Design review of the part built by this model. Coordinates are the model's own, in mm. A direction names the side the tool comes from. Round coordinates to 2 decimals unless told otherwise and drop trailing zeros. Order: outer loops, then holes, each group sorted by start corner. A loop starts at its lowest first (then second) coordinate and runs counter-clockwise, first axis right, second up. Notation, with made-up numbers: (8, 73.25) - (54, 73.25) arc R25 cw to (54, 103.25) - close; hole circle Ø8 at (-36, 74). An arc over 180 degrees is marked (long way). Use CSV: the item, a comma, the result in double quotes.
Autodesk Inventor part; units mm, degrees
ref_plane "XZ Plane" through (0, 0, 0) normal (0, 1, 0) x (-1, 0, 0)
ref_plane "XY Plane" through (0, 0, 0) normal (0, 0, 1) x (1, 0, 0)
sketch "Sketch1" plane through (0, 0, 0) normal (0, 1, 0) x (-1, 0, 0)
  circle A0 centre (0, 0) radius 17.5
  arc A1 (-20.1304, -3.875) -> (-20.1304, 3.875) centre (0, 0) ccw
  line L0 (-20.5, -3.875) -> (-20.5, -13.4374) construction
  line L1 (-20.5, -13.4374) -> (-20.5, 14.7091) construction
  line L2 (-47.5, 3.875) -> (-47.5, -3.875)
  line L3 (-47.5, -3.875) -> (-20.1304, -3.875)
  line L4 (0, 0) -> (-47.4736, 0) construction
  line L5 (-47.5, 3.875) -> (-20.1304, 3.875)
  dimension "d0" = 35
  dimension "d1" = 3
  dimension "d4" = 27
extrude "Extrusion1" add sketch "Sketch1" along normal blind 40
sketch "Sketch2" plane through (20.1304, 0, 3.875) normal (0, 0, 1) x (1, 0, 0)
  line L0 (27.3696, 0) -> (27.3696, 40)
  line L1 (2, 40) -> (27.3696, 40)
  line L2 (17.5718, 20.8426) -> (6, 0)
  line L3 (27.3696, 0) -> (0, 0)
  line L4 (27.3696, 0) -> (27.3696, 40)
  line L5 (6, 0) -> (27.3696, 0)
  line L6 (27.3696, 0) -> (27.3696, 28)
  line L7 (0, 0) -> (0, 40)
  arc A0 (17.5718, 20.8426) -> (12.9208, 36.4588) centre (17, 29.173) ccw
  line L8 (12.9208, 36.4588) -> (0, 40)
  circle A1 centre (17, 29.173) radius 3.825
  line L9 (0, 40) -> (27.3696, 40)
  line L10 (27.3696, 0) -> (6, 0)
  point P0 (-20.1304, 0)
  dimension "d10" = 6
  dimension "d14" = 16.7
  dimension "d15" = 17
  dimension "d16" = 7.65
extrude "Extrusion2" cut sketch "Sketch2" against normal blind 40 contours L3 L2 A0 L8 L9 L1 L0 | A1
ref_plane "Work Plane1" through (-12, 0, 0) normal (1, 0, 0) x (0, 1, 0)
split "Split1" plane through (-12, 0, 0) removes the side toward (-1, 0, 0)
chamfer "Chamfer1" distance 1.5 angle 45 1 edges at (17.5, 0, 0)
chamfer "Chamfer2" distance 1.5 angle 45 1 edges at (17.5, 40, 0)
fillet "Fillet1" radius 6 1 edges at (20.1304, 20, 3.875)
fillet "Fillet2" radius 6 1 edges at (20.1304, 20, -3.875)
fillet "Fillet3" radius 6 1 edges at (26.1304, 0, 0)
fillet "Fillet4" radius 3 2 edges at (-12, 20, -16.6208) (-12, 20, 16.6208)
fillet_without_effect "Fillet5"
fillet "Fillet6" radius 3 2 edges at (-12, 20, -12.7377) (-12, 20, 12.7377)
properties part number "Radio Mic Holder"
1) We need section C-C (y = 15.5). Give the boundary of the cut face in (x, z) (3 decimals), then the cut area to 3 significant figures.
Data:
outline,"(-12, -15.008) arc R3 ccw to (-10.543, -17.581) arc R20.5 ccw to (19.023, -7.639) arc R6 cw to (24.591, -3.875) - (34.736, -3.875) - (34.736, 3.875) - (24.591, 3.875) arc R6 cw to (19.023, 7.639) arc R20.5 ccw to (-10.543, 17.581) arc R3 ccw to (-12, 15.008) arc R3 ccw to (-8.964, 15.03) arc R17.5 cw (long way) to (-8.964, -15.03) arc R3 ccw to start"
area,"370 mm2"
2) Insertion check: pin 1 Ø6.5 at (x, y) = (33.5, 23.5) entering from -Z (3 decimals); pin 2 Ø5 at (x, y) = (9.5, 24.5) entering from -Z; pin 3 Ø10.5 at (x, y) = (34, 16.5) entering from +Z (3 decimals); pin 4 Ø4 at (y, z) = (12, 13.5) entering from -X. Each pin has a flat end and moves straight along its axis. Give the tip position at first contact, or say it passes through.
Data:
pin 1,"stops at z = -3.875"
pin 2,"stops at z = -19.27"
pin 3,"stops at z = 3.875"
pin 4,"stops at x = -12"
3) We need section A-A (x = 0). Give the boundary of the cut face in (y, z).
Data:
outline,"(0, -20.5) - (40, -20.5) - (40, -19) - (38.5, -17.5) - (1.5, -17.5) - (0, -19) - close; (0, 19) - (1.5, 17.5) - (38.5, 17.5) - (40, 19) - (40, 20.5) - (0, 20.5) - close"
4) For faces 1 (the face through (-10.457, 20.28, 14.607)), 2 (the face through (33, 24, -3.875)), 3 (the face through (33, 24, 3.875)), 4 (the face through (-11.62, 19.72, -16.47)), list the 3-axis set-ups (+Z, -Z, +X, -X, +Y, -Y) from which the entire face can be reached by the end or side of a thin tool; tool diameter is ignored.
Data:
face 1,"+Y, -Y"
face 2,"-Z, +X, +Y, -Y"
face 3,"+Z, +X, +Y, -Y"
face 4,"-Z, -X, +Y, -Y"
5) To check wall thickness, follow L1, parallel to Z at x = 0, y = 27; L2, parallel to Z at x = 6, y = 5; L3, parallel to X at y = 27, z = 16. State the ranges of each line that lie inside material, in increasing order. Write a range as from..to.
Data:
L1,"z = -20.5..-17.5, 17.5..20.5"
L2,"z = -19.6..-16.44, 16.44..19.6"
L3,"x = -11.83..-7.09, 7.09..12.82"
6) We need section B-B (z = 0). Give the boundary of the cut face in (x, y) (3 decimals), then the cut area to 3 significant figures.
Data:
outline,"(17.5, 1.5) - (19, 0) - (22.599, 0) arc R6 ccw to (27.845, 3.088) - (37.702, 20.843) arc R8.35 ccw (long way) to (33.051, 36.459) - (20.13, 40) - (19, 40) - (17.5, 38.5) - close; hole circle Ø7.65 at (37.13, 29.173)"
area,"701 mm2"
7) We need section D-D (x = 32). Give the boundary of the cut face in (y, z) (3 decimals), then the cut area to 3 significant figures.
Data:
outline,"(10.572, -3.875) - (36.747, -3.875) - (36.747, 3.875) - (10.572, 3.875) - close"
area,"203 mm2"
8) The part is to be moulded in two halves that separate along X. For faces 5 (the face through (-10.501, 20.28, -14.607)), 6 (the face through (21.27, 20.28, 4.88)), 7 (the face through (26.7, 38.2, 0.1)), 8 (the face through (19.6, 40, 0.1)), say which applies: +X half, -X half, draft (parallel to the pull), parting line (faces both ways), or undercut.
Data:
face 5,"undercut"
face 6,"+X half"
face 7,"undercut"
face 8,"draft"
